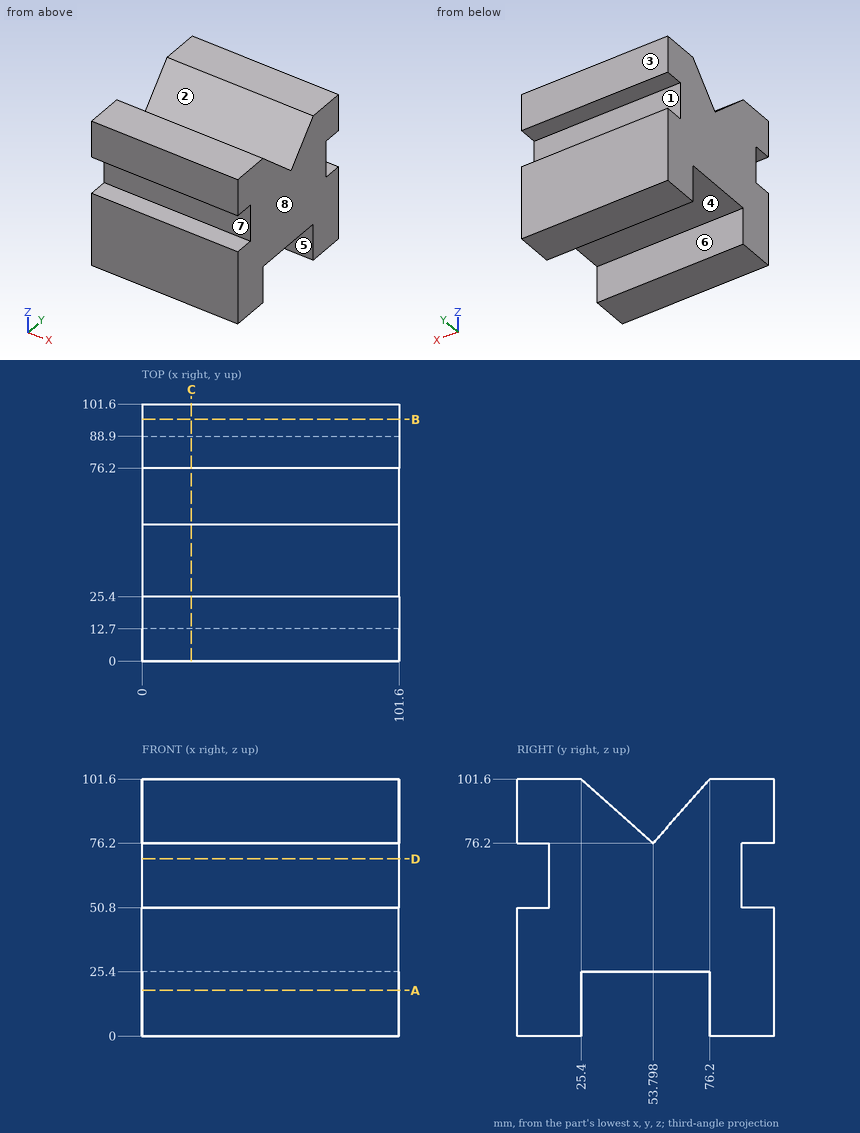
Answer from the drawing. Dimensions are ordinates in mm from the lowest x, y and z of the part. A direction names the side the tool comes from. Round coordinates to 2 decimals unless told otherwise and drop trailing zeros. Write each loop counter-clockwise with the first axis right and the second up, starting at its lowest first coordinate (ties: lowest second). Pieces come first, ordered by that corner, then holes.
1. Straight lines are drawn through the part: L1, parallel to Z at x = 67.5, y = 94; L2, parallel to Y at x = 60, z = 12.5; L3, parallel to Y at x = 78, z = 68.5. For each, find the intervals that lie inside material, in ascending order.
2. The part is cut by section A-A, the plane z = 18. Determine the outline of the cut face in (x, y), then the cut area to 3 significant figures.
3. Determine the mould class of the marked faces 5, 6, 7 and 8 for opening direction Y: pulls with the +Y half, pulls with the -Y half, needs draft (parallel to the pull), parting line crosses it, or undercut.
4. Given pin 1 Ø12 at (x, y) = (22, 45.5) entering from -Z; pin 2 Ø7.5 at (x, z) = (53, 68.5) entering from +Y; pin 3 Ø10 at (x, y) = (63, 95.5) entering from -Z, each flat-ended and moving along its own axis, determine where each tip first touches the part or whether it passes through.
5. The part is cut by section C-C, the plane x = 19.5. Determine the outline of the cut face in (y, z), then the cut area to 3 significant figures.
6. The part is cut by section D-D, the plane z = 70. Determine the outline of the cut face in (x, y).
7. Which of the six approach directions +Z, -Z, +X, -X, +Y, -Y give full straight-line access (tool end or side, diameter ignored) to the marked faces 1, 2, 3 and 4?
8. The part is cut by section B-B, the plane y = 95.5. Determine the outline of the cut face in (x, z).
Values:
1. L1: z = 0 to 50.8, 76.2 to 101.6
1. L2: y = 0 to 25.4, 76.2 to 101.6
1. L3: y = 12.7 to 88.9
2. outline: (0, 0) - (101.6, 0) - (101.6, 25.4) - (0, 25.4) - close; (0, 76.2) - (101.6, 76.2) - (101.6, 101.6) - (0, 101.6) - close
2. area: 5,160 mm2
3. face 5: undercut
3. face 6: undercut
3. face 7: pulls with the -Y half
3. face 8: needs draft
4. pin 1: stops at z = 25.4
4. pin 2: stops at y = 88.9
4. pin 3: stops at z = 0
5. outline: (0, 0) - (25.4, 0) - (25.4, 25.4) - (76.2, 25.4) - (76.2, 0) - (101.6, 0) - (101.6, 50.8) - (88.9, 50.8) - (88.9, 76.2) - (101.6, 76.2) - (101.6, 101.6) - (76.2, 101.6) - (53.8, 76.2) - (25.4, 101.6) - (0, 101.6) - (0, 76.2) - (12.7, 76.2) - (12.7, 50.8) - (0, 50.8) - close
5. area: 7,740 mm2
6. outline: (0, 12.7) - (101.6, 12.7) - (101.6, 88.9) - (0, 88.9) - close
7. face 1: +X, -X, +Y
7. face 2: +Z, +X, -X
7. face 3: +Z, -Z, +X, -X, +Y
7. face 4: -Z, +X, -X
8. outline: (0, 0) - (101.6, 0) - (101.6, 50.8) - (0, 50.8) - close; (0, 76.2) - (101.6, 76.2) - (101.6, 101.6) - (0, 101.6) - close
